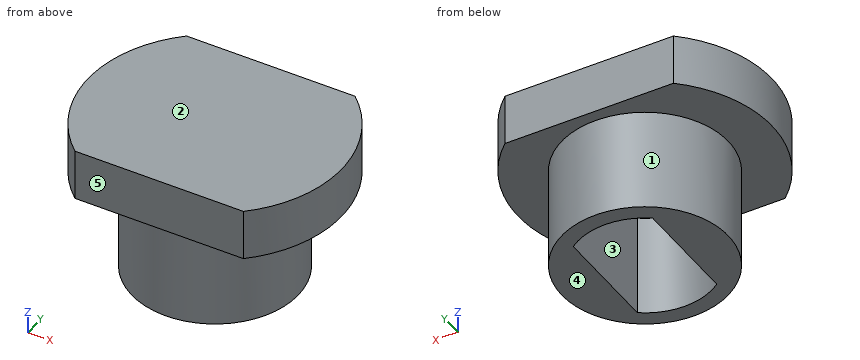
from build123d import *

# Parameters (mm, degrees)
F0_R     = 6.5
F1_DEPTH = 8
F3_DEPTH = 8
F4_R     = 9.9
F5_DEPTH = 4
F7_DEPTH = 4


with BuildPart() as f1:
    # F0 (on Top) → F1 (new body)
    with BuildSketch(Plane.XY):
        Circle(F0_R)
    extrude(amount=F1_DEPTH)

    # F2 (on face) → F3 (cut, through all)
    with BuildSketch(Plane.XY.offset(8)):
        with BuildLine():
            ThreePointArc((3.1, 4.25), (0, 5.260466), (-3.1, 4.25))
            Line((-3.1, 4.25), (-3.1, -4.25))
            ThreePointArc((-3.1, -4.25), (0, -5.260466), (3.1, -4.25))
            Line((3.1, -4.25), (3.1, 4.25))
        make_face()
    extrude(amount=-F3_DEPTH, mode=Mode.SUBTRACT)

    # F4 (on face) → F5 (join)
    with BuildSketch(Plane.XY.offset(8)):
        Circle(F4_R)
    extrude(amount=F5_DEPTH)

    # F6 (on face) → F7 (cut, through all)
    with BuildSketch(Plane.XY.offset(12)):
        with BuildLine():
            ThreePointArc((6.576473, 7.4), (0, 9.9), (-6.576473, 7.4))
            Line((-6.576473, 7.4), (6.576473, 7.4))
        make_face()
        with BuildLine():
            Line((6.576473, -7.4), (-6.576473, -7.4))
            ThreePointArc((-6.576473, -7.4), (0, -9.9), (6.576473, -7.4))
        make_face()
    extrude(amount=-F7_DEPTH, mode=Mode.SUBTRACT)


solid = f1.part
Can you work these out from the model? Positions are in its coordinate system, mm. Face numbers are marked on the shaded views. A direction names the side the tool comes from. Give positions to 0.01 mm unless a question says otherwise; leave off trailing zeros. Loops run counter-clockwise (first coordinate to the right, second up) from the corner with the lowest first, then second, coordinate; pieces in that order, holes last. Notation, with made-up numbers: (81, 51.5) - (137, 51.5) arc R24 ccw to (137, 67.5) - close; hole circle Ø8 at (38.5, 1.5). An arc over 180 degrees is marked (long way). Return JSON: item names as keys, results as strings.
1. I want a section at B-B on z = 3. Please give me the cut outline in (x, y).
Output values:
{"outline": "circle Ø13 at (0, 0); hole (-3.1, -4.25) arc R5.26 ccw to (3.1, -4.25) - (3.1, 4.25) arc R5.26 ccw to (-3.1, 4.25) - close"}
2. I want a section at D-D on z = 8.25. Please give me the cut outline in (x, y), and give its area (3 significant figures).
Output values:
{"outline": "(-6.58, -7.4) - (6.58, -7.4) arc R9.9 ccw to (6.58, 7.4) - (-6.58, 7.4) arc R9.9 ccw to start", "area": "263 mm²"}
3. I want a section at A-A on y = 0. Please give me the cut outline in (x, z), and give its area (3 significant figures).
Output values:
{"outline": "(-9.9, 8) - (-6.5, 8) - (-6.5, 0) - (-3.1, 0) - (-3.1, 8) - (3.1, 8) - (3.1, 0) - (6.5, 0) - (6.5, 8) - (9.9, 8) - (9.9, 12) - (-9.9, 12) - close", "area": "134 mm²"}
4. If I drill on line 1 (Z direction, x = 6.5, y = -6); line 2 (X direction, y = -1.5, z = 4.25); line 3 (X direction, y = 0.5, z = 6.75), over which ranges is the centre line in solid material (lowest first)?
Output values:
{"line 1": "z = 8 to 12", "line 2": "x = -6.32 to -3.1, 3.1 to 6.32", "line 3": "x = -6.48 to -3.1, 3.1 to 6.48"}
5. For the marked faces 1 and 2, which set-ups out of +Z, -Z, +X, -X, +Y, -Y let a thin tool reach every point of the face, with its end or its side?
Output values:
{"face 1": "-Z", "face 2": "+Z, +X, -X, +Y, -Y"}
6. We'd pull the mould along Y, two halves only. Please class the marked faces 3, 4 and 5: +Y half, -Y half, draft (parallel to the pull), parting line (faces both ways), or undercut.
Output values:
{"face 3": "undercut", "face 4": "draft", "face 5": "-Y half"}
7. I'm going to push flat-ended pins straight in: pin 1 Ø2 at (y, z) = (2, 8) entering from +X; pin 2 Ø2.5 at (y, z) = (1, 5.5) entering from +X; pin 3 Ø1.5 at (y, z) = (-5.5, 3.5) entering from +X. Where does each tip first touch, or does it pass through?
Output values:
{"pin 1": "stops at x = 9.85", "pin 2": "stops at x = 6.5", "pin 3": "stops at x = 4.44"}
8. I want a section at C-C on x = 0. Please give me the cut outline in (y, z), and give its area (3 significant figures).
Output values:
{"outline": "(-7.4, 8) - (-6.5, 8) - (-6.5, 0) - (-5.26, 0) - (-5.26, 8) - (5.26, 8) - (5.26, 0) - (6.5, 0) - (6.5, 8) - (7.4, 8) - (7.4, 12) - (-7.4, 12) - close", "area": "79.0 mm²"}
